from build123d import *

# Parameters (mm, degrees)
SKETCH1_R           = 2.5
SKETCH1_R_2         = 38.5
BOSS_EXTRUDE1_DEPTH = 4
FILLET1_R           = 3
EXTRUDE_THIN1_DEPTH = 4
FILLET2_R           = 10
FILLET3_R           = 4
FILLET4_R           = 1
SKETCH3_R           = 64.024386015
CUT_EXTRUDE1_DEPTH  = 10
FILLET5_R           = 5
FILLET6_DEPTH       = 4


with BuildPart() as part:
    # Sketch1 → Boss-Extrude1 (new body)
    with BuildSketch(Plane(origin=(0, 0, 0), x_dir=(1, 0, 0), z_dir=(0, 1, 0))):
        with BuildLine():
            ThreePointArc((30.517857143, 5.446135824), (21.920310217, 21.920310217), (5.446135824, 30.517857143))
            ThreePointArc((5.446135824, 30.517857143), (0, 34), (-5.446135824, 30.517857143))
            ThreePointArc((-5.446135824, 30.517857143), (-20.638377106, 23.131307581), (-29.702130488, 8.876003857))
            ThreePointArc((-29.702130488, 8.876003857), (-31.212792428, 6.764161745), (-33.701829376, 6.02478926))
            ThreePointArc((-33.701829376, 6.02478926), (-54.791240945, -1.442417701), (-64.849322602, -21.426347583))
            ThreePointArc((-64.849322602, -21.426347583), (-66.120648036, -24.027926305), (-68.814456997, -25.089940189))
            ThreePointArc((-68.814456997, -25.089940189), (-99.348502757, -99.348502757), (-25.089940189, -68.814456997))
            ThreePointArc((-25.089940189, -68.814456997), (-24.027926305, -66.120648036), (-21.426347583, -64.849322602))
            ThreePointArc((-21.426347583, -64.849322602), (-1.442417701, -54.791240945), (6.02478926, -33.701829376))
            ThreePointArc((6.02478926, -33.701829376), (6.764161745, -31.212792428), (8.876003857, -29.702130488))
            ThreePointArc((8.876003857, -29.702130488), (23.131307581, -20.638377106), (30.517857143, -5.446135824))
            ThreePointArc((30.517857143, -5.446135824), (34, 0), (30.517857143, 5.446135824))
        make_face()
        with Locations(Location((0, 28, 0), (0, 0, 270))):
            Circle(SKETCH1_R, mode=Mode.SUBTRACT)
        with Locations(Location((28, 0, 0), (0, 0, 270))):
            Circle(SKETCH1_R, mode=Mode.SUBTRACT)
        with Locations(Location((0, -28, 0), (0, 0, 270))):
            Circle(SKETCH1_R, mode=Mode.SUBTRACT)
        with Locations(Location((-28, 0, 0), (0, 0, 270))):
            Circle(SKETCH1_R, mode=Mode.SUBTRACT)
        with Locations(Location((-68.589357775, -68.589357775, 0), (0, 0, 270))):
            Circle(SKETCH1_R_2, mode=Mode.SUBTRACT)
        with BuildLine():
            ThreePointArc((-24.517857143, -4.886172441), (-17.67766953, -17.67766953), (-4.886172441, -24.517857143))
            ThreePointArc((-4.886172441, -24.517857143), (0, -22), (4.886172441, -24.517857143))
            ThreePointArc((4.886172441, -24.517857143), (17.67766953, -17.67766953), (24.517857143, -4.886172441))
            ThreePointArc((24.517857143, -4.886172441), (22, 0), (24.517857143, 4.886172441))
            ThreePointArc((24.517857143, 4.886172441), (17.67766953, 17.67766953), (4.886172441, 24.517857143))
            ThreePointArc((4.886172441, 24.517857143), (0, 22), (-4.886172441, 24.517857143))
            ThreePointArc((-4.886172441, 24.517857143), (-17.67766953, 17.67766953), (-24.517857143, 4.886172441))
            ThreePointArc((-24.517857143, 4.886172441), (-22, 0), (-24.517857143, -4.886172441))
        make_face(mode=Mode.SUBTRACT)
        with BuildLine():
            ThreePointArc((-50.542739629, -29.009444012), (-37.830212793, -37.830212793), (-29.009444012, -50.542739629))
            ThreePointArc((-29.009444012, -50.542739629), (-27.701648922, -52.133357655), (-25.775886095, -52.862625259))
            ThreePointArc((-25.775886095, -52.862625259), (-11.221079312, -47.683495854), (-6.041949907, -33.128689072))
            ThreePointArc((-6.041949907, -33.128689072), (-6.938958159, -30.985310284), (-8.876003857, -29.702130488))
            ThreePointArc((-8.876003857, -29.702130488), (-21.920310217, -21.920310217), (-29.702130488, -8.876003857))
            ThreePointArc((-29.702130488, -8.876003857), (-30.985310284, -6.938958159), (-33.128689072, -6.041949907))
            ThreePointArc((-33.128689072, -6.041949907), (-47.683495854, -11.221079312), (-52.862625259, -25.775886095))
            ThreePointArc((-52.862625259, -25.775886095), (-52.133357655, -27.701648922), (-50.542739629, -29.009444012))
        make_face(mode=Mode.SUBTRACT)
    extrude(amount=BOSS_EXTRUDE1_DEPTH)

    # Fillet1
    fillet1_edges = [part.edges().sort_by_distance(p)[0] for p in [
        (5.446135824, 2, -30.517857143),
        (30.517857143, 2, -5.446135824),
        (30.517857143, 2, 5.446135824),
        (-5.446135824, 2, -30.517857143),
        (24.517857143, 2, -4.886172441),
        (4.886172441, 2, -24.517857143),
        (-4.886172441, 2, -24.517857143),
        (-24.517857143, 2, -4.886172441),
        (-24.517857143, 2, 4.886172441),
        (-4.886172441, 2, 24.517857143),
        (4.886172441, 2, 24.517857143),
        (24.517857143, 2, 4.886172441),
    ]]
    fillet(fillet1_edges, radius=FILLET1_R)

    # Sketch2 → Extrude-Thin1 (add)
    with BuildSketch(Plane(origin=(0, 4, 0), x_dir=(1, 0, 0), z_dir=(0, 1, 0))):
        with BuildLine():
            Line((-32.237774047, -50.35980695), (-29.529509942, -48.389301254))
            ThreePointArc((-29.529509942, -48.389301254), (-28.482745443, -48.04910113), (-27.43634696, -48.390425395))
            ThreePointArc((-27.43634696, -48.390425395), (-9.798865492, -43.800084833), (-17.778530097, -27.414819141))
            Line((-17.778530097, -27.414819141), (-39.072120949, -22.36364217))
            ThreePointArc((-39.072120949, -22.36364217), (-40.242802597, -19.82149687), (-37.49426164, -19.293746119))
            ThreePointArc((-37.49426164, -19.293746119), (-30.900503465, -22.135181432), (-23.882232512, -20.620165146))
            Line((-23.882232512, -20.620165146), (-21.436410838, -19.212144584))
            Line((-21.436410838, -19.212144584), (-26.425576805, -10.545644543))
            Line((-26.425576805, -10.545644543), (-28.871398479, -11.953665105))
            ThreePointArc((-28.871398479, -11.953665105), (-29.930650966, -12.182323243), (-30.925832655, -11.753471545))
            ThreePointArc((-30.925832655, -11.753471545), (-49.13679313, -15.250180603), (-41.380227899, -32.093628928))
            Line((-41.380227899, -32.093628928), (-20.086637047, -37.144805898))
            ThreePointArc((-20.086637047, -37.144805898), (-18.882283492, -39.617798683), (-21.5442705, -40.310608876))
            ThreePointArc((-21.5442705, -40.310608876), (-28.477374908, -38.049102572), (-35.412904416, -40.303160675))
            Line((-35.412904416, -40.303160675), (-38.121168521, -42.273666371))
            Line((-38.121168521, -42.273666371), (-32.237774047, -50.35980695))
        make_face()
    extrude(amount=-EXTRUDE_THIN1_DEPTH)

    # Fillet2
    fillet2_edges = [part.edges().sort_by_distance(p)[0] for p in [
        (-23.394596499, 2, 20.339440864),
    ]]
    fillet(fillet2_edges, radius=FILLET2_R)

    # Fillet3
    # the kernel refuses this fillet: 4 mm, written as the material it adds along each edge
    with BuildSketch(Plane(origin=(-28.654487562, 4, 11.828792947), x_dir=(-0.3625938431900147, 0, -0.9319472650749584), z_dir=(0, -1, 0))) as fillet3_piece_1:
        with BuildLine():
            CenterArc((1.34953067, -3.999163717), FILLET3_R, 91.171633345, 19.12091028)
            Line((-0.037723703, -0.247427412), (-0.065468791, -0.172392686))
            ThreePointArc((-0.065468791, -0.172392686), (-0.097947947, -0.111655946), (-0.079086095, 0.01205776))
            Line((-0.079086095, 0.01205776), (0.001635795, 0.079983274))
            ThreePointArc((0.001635795, 0.079983274), (0.633870466, 0.07351881), (1.266105138, 0.079983274))
            Line((1.266105138, 0.079983274), (1.267740932, 0))
        make_face()
    extrude(amount=4)
    with BuildSketch(Plane(origin=(-29.917309098, 4, 48.671460016), x_dir=(0.8086140578930259, 0, -0.5883394474092097), z_dir=(0, -1, 0))) as fillet3_piece_2:
        with BuildLine():
            CenterArc((3.628329627, 2.4668618), FILLET3_R, 191.061242736, 27.015431221)
            Line((-0.29736105, 1.69942926), (-0.375874864, 1.684080609))
            ThreePointArc((-0.375874864, 1.684080609), (-0.219057332, 0.837400307), (-0.079060684, -0.012223264))
            Line((-0.079060684, -0.012223264), (0, -0.08))
            ThreePointArc((0, -0.08), (0.23979249, -0.08), (0.416610086, -0.049337236))
            Line((0.416610086, -0.049337236), (0.479584979, 0))
        make_face()
    extrude(amount=4)

    # Fillet4
    fillet4_edges = [part.edges().sort_by_distance(p)[0] for p in [
        (-28.871398479, 2, 11.953665105),
        (-29.529509942, 2, 48.389301254),
    ]]
    fillet(fillet4_edges, radius=FILLET4_R)

    # Sketch3 → Cut-Extrude1 (cut)
    with BuildSketch(Plane(origin=(0, 4, 0), x_dir=(1, 0, 0), z_dir=(0, 1, 0))):
        with Locations((-98.613587898, -92.689059133)):
            Circle(SKETCH3_R)
    extrude(amount=-CUT_EXTRUDE1_DEPTH, mode=Mode.SUBTRACT)

    # Fillet5
    # the kernel refuses this fillet: 5 mm, written as the material it takes off along each edge
    with BuildSketch(Plane(origin=(-34.665740184, 37.003417613, 95.818720043), x_dir=(0.5003791783842261, 0, -0.865806374335236), z_dir=(0, -1, 0))) as fillet5_piece_1:
        with BuildLine():
            CenterArc((12.44266779, -4.94210233), FILLET5_R, 81.272233046, 93.723124761)
            Line((7.461729623, -4.505920051), (7.36211086, -4.497196406))
            ThreePointArc((7.36211086, -4.497196406), (3.755943973, -2.211429345), (-0.045745837, -0.088923104))
            Line((-0.045745837, -0.088923104), (-0.015173985, 0.098842047))
            ThreePointArc((-0.015173985, 0.098842047), (6.600683523, 0.603709729), (13.21654103, 0.098842047))
            Line((13.21654103, 0.098842047), (13.201367045, 0))
        make_face()
    extrude(amount=70.006835226, mode=Mode.SUBTRACT)
    with BuildSketch(Plane(origin=(-87.835142464, 37.003417613, 29.578464787), x_dir=(0.9719808160710193, 0, 0.23506019056810815), z_dir=(0, -1, 0))) as fillet5_piece_2:
        with BuildLine():
            CenterArc((13.205988808, -2.20141245), FILLET5_R, 153.878093502, 93.723124761)
            Line((11.300735218, -6.82418313), (11.262630146, -6.916638544))
            ThreePointArc((11.262630146, -6.916638544), (5.338291917, -3.928883786), (-0.064083773, -0.076767636))
            Line((-0.064083773, -0.076767636), (0.006807322, 0.099768033))
            ThreePointArc((0.006807322, 0.099768033), (4.358346145, -0.048515583), (8.62690636, 0.044028249))
            Line((8.62690636, 0.044028249), (8.71669229, 0))
        make_face()
    extrude(amount=70.006835226, mode=Mode.SUBTRACT)

    # Fillet6: read off the stored shape, not the designer's step
    # Fillet6 outline → Fillet6 (add)
    with BuildSketch(Plane(origin=(0, 0, 0), x_dir=(1, 0, 0), z_dir=(0, 1, 0))):
        with BuildLine():
            ThreePointArc((-30.985608924, -38.317908864), (-35.637111816, -38.221540359), (-39.741582528, -36.03085868))
            ThreePointArc((-39.741582528, -36.03085868), (-37.541405134, -38.121757988), (-35.492388329, -40.36099237))
            Line((-35.492388329, -40.36099237), (-35.412904416, -40.303160675))
            ThreePointArc((-35.412904416, -40.303160675), (-33.302598309, -39.080073338), (-30.985608924, -38.317908864))
        make_face()
    extrude(amount=FILLET6_DEPTH)


solid = part.part
Can you work these out from the model? Positions are in its coordinate system, mm. A direction names the side the tool comes from. Coordinates: 2 decimals unless noted, no trailing zeros. Loops run counter-clockwise (first coordinate to the right, second up) from the corner with the lowest first, then second, coordinate; pieces in that order, holes last. Notation, with made-up numbers: (88.5, -12) - (120.5, -12) arc R22 ccw to (120.5, 16) - close; hole circle Ø3 at (-19.5, 74.25). An arc over 180 degrees is marked (long way). Put each result on its own line as item: value. Start each with the question number.
Item 1: Suppose I cut it at A-A (x = 0). Please give me the cut outline in (y, z).
Item 2: If we mould it in two halves opening along Z, with no side actions, what happens to faces 1 (the face through (0.1, 2, -30.5)), 2 (the face through (-25.88, 1.97, 76.85)), 3 (the face through (-20.94, 1.97, -22.86)), 4 (the face through (-14.407, 1.972, 27.449))? For each: +Z half, -Z half, draft (parallel to the pull), parting line (faces both ways), or undercut.
Item 3: Suppose I cut it at B-B (x = 28). Please give me the cut outline in (y, z).
Item 4: Which directions (+Z, -Z, +X, -X, +Y, -Y) give clear straight access to the entire face, cutting with the end or side of a thin tool? Please do faces 5 (the face through (-23, 4, 27)), 6 (the face through (-30.882, 2.028, 34.584)).
Item 5: Suppose I cut it at C-C (z = 0). Please give me the cut outline in (x, y), and give its area (3 significant figures).
Item 6: Suppose I cut it at D-D (z = -28). Please give me the cut outline in (x, y).
Item 7: If I drill on line 1 along X through (y, z) = (2.4, 49.5); line 2 along Z through (x, y) = (23, 0.35); line 3 along Z through (x, y) = (-36, 1.65), over which ranges is the centre line in solid material (lowest first)?
Item 8: For pin 1 (1.5 mm diameter, centred on x = 19.5, y = 0.5, fed in from -Z); pin 2 (1 mm diameter, centred on y = 1.5, z = 2, fed in from -X); pin 3 (1 mm diameter, centred on x = 17, y = 1, fed in from -Z), each with a flat end and sliding along its axis, tell me the tip position at first contact or that it passes through.
Here are the results:
1. outline: (0, -34) - (4, -34) - (4, -30.5) - (0, -30.5) - close; (0, -25.5) - (4, -25.5) - (4, -22) - (0, -22) - close; (0, 22) - (4, 22) - (4, 25.5) - (0, 25.5) - close; (0, 30.5) - (4, 30.5) - (4, 53.02) - (0, 53.02) - close
2. face 1: undercut
2. face 2: +Z half
2. face 3: -Z half
2. face 4: undercut
3. outline: (0, -13.3) - (4, -13.3) - (4, -2.5) - (0, -2.5) - close; (0, 2.5) - (4, 2.5) - (4, 13.3) - (0, 13.3) - close
4. face 5: +Z, -Z, +X, -X, +Y
4. face 6: +Y, -Y
5. outline: (-53.02, 0) - (-30.5, 0) - (-30.5, 4) - (-53.02, 4) - close; (-25.5, 0) - (-22, 0) - (-22, 4) - (-25.5, 4) - close; (22, 0) - (25.5, 0) - (25.5, 4) - (22, 4) - close; (30.5, 0) - (34, 0) - (34, 4) - (30.5, 4) - close
5. area: 132 mm²
6. outline: (-13.3, 0) - (-2.5, 0) - (-2.5, 4) - (-13.3, 4) - close; (2.5, 0) - (13.3, 0) - (13.3, 4) - (2.5, 4) - close
7. line 1: -35.16 to -29.41, -25.58 to -15.42, -13.34 to 2.29
7. line 2: -20.78 to -9.8, -3.32 to 3.32, 9.8 to 20.78
7. line 3: -6.03 to 5.98, 9.16 to 20.4, 23.09 to 33.37, 38.12 to 48.09
8. pin 1: z = -24.69
8. pin 2: x = -55.93
8. pin 3: z = -26.24
